from build123d import *

# Parameters (mm, degrees)
SKETCH1_R           = 10.5
SKETCH1_R_2         = 9
BOSS_EXTRUDE1_DEPTH = 15
CUT_EXTRUDE1_START  = 9.5
CUT_EXTRUDE1_DEPTH  = 2


with BuildPart() as part:
    # Sketch1 → Boss-Extrude1 (new body, symmetric)
    with BuildSketch(Plane(origin=(0, 0, 0), x_dir=(1, 0, 0), z_dir=(0, 1, 0))):
        Circle(SKETCH1_R)
        Circle(SKETCH1_R_2, mode=Mode.SUBTRACT)
    extrude(amount=BOSS_EXTRUDE1_DEPTH, both=True)

    # Sketch2 → Cut-Extrude1 (cut)
    with BuildSketch(Plane(origin=(0, 0, 0), x_dir=(0, 0, -1), z_dir=(1, 0, 0)).offset(CUT_EXTRUDE1_START)):
        with BuildLine():
            ThreePointArc((-2.374052789, 1.874699538), (-1.648827359, 2.536137485), (-0.75, 2.93055029))
            Line((-0.75, 2.93055029), (-0.75, 5))
            add(Edge.make_bspline(
                [(-0.75, 5), (-0.968656254, 3.654443702), (-2.374052789, 1.874699538)],
                knots=[0, 0, 0, 1, 1, 1], degree=2))
        make_face()
        with BuildLine():
            ThreePointArc((-2.374052789, -1.874699538), (-1.648827359, -2.536137485), (-0.75, -2.93055029))
            Line((-0.75, -2.93055029), (-0.75, 2.93055029))
            ThreePointArc((-0.75, 2.93055029), (-1.648827359, 2.536137485), (-2.374052789, 1.874699538))
            ThreePointArc((-2.374052789, 1.874699538), (-3.025, 0), (-2.374052789, -1.874699538))
        make_face()
        with BuildLine():
            Line((0.75, 2.93055029), (0.75, -2.93055029))
            ThreePointArc((0.75, -2.93055029), (1.648827359, -2.536137485), (2.374052789, -1.874699538))
            ThreePointArc((2.374052789, -1.874699538), (2.857633171, -0.992248788), (3.025, 0))
            ThreePointArc((3.025, 0), (2.857633171, 0.992248788), (2.374052789, 1.874699538))
            ThreePointArc((2.374052789, 1.874699538), (1.648827359, 2.536137485), (0.75, 2.93055029))
        make_face()
        with BuildLine():
            Line((0.75, 5), (0.75, 2.93055029))
            ThreePointArc((0.75, 2.93055029), (1.648827359, 2.536137485), (2.374052789, 1.874699538))
            add(Edge.make_bspline(
                [(0.75, 5), (0.968656254, 3.654443702), (2.374052789, 1.874699538)],
                knots=[0, 0, 0, 1, 1, 1], degree=2))
        make_face()
        with BuildLine():
            Line((0.75, -2.93055029), (0.75, -5))
            add(Edge.make_bspline(
                [(0.75, -5), (0.968656254, -3.654443702), (2.374052789, -1.874699538)],
                knots=[0, 0, 0, 1, 1, 1], degree=2))
            ThreePointArc((2.374052789, -1.874699538), (1.648827359, -2.536137485), (0.75, -2.93055029))
        make_face()
        with BuildLine():
            Line((-0.75, -5), (0.75, -5))
            Line((0.75, -5), (0.75, -2.93055029))
            ThreePointArc((0.75, -2.93055029), (0, -3.025), (-0.75, -2.93055029))
            Line((-0.75, -2.93055029), (-0.75, -5))
        make_face()
        with BuildLine():
            add(Edge.make_bspline(
                [(-0.75, -5), (-0.968656254, -3.654443702), (-2.374052789, -1.874699538)],
                knots=[0, 0, 0, 1, 1, 1], degree=2))
            Line((-0.75, -5), (-0.75, -2.93055029))
            ThreePointArc((-0.75, -2.93055029), (-1.648827359, -2.536137485), (-2.374052789, -1.874699538))
        make_face()
        with BuildLine():
            ThreePointArc((-0.75, 2.93055029), (0, 3.025), (0.75, 2.93055029))
            Line((0.75, 2.93055029), (0.75, 5))
            Line((0.75, 5), (-0.75, 5))
            Line((-0.75, 5), (-0.75, 2.93055029))
        make_face()
        with BuildLine():
            ThreePointArc((-0.75, -2.93055029), (0, -3.025), (0.75, -2.93055029))
            Line((0.75, -2.93055029), (0.75, 2.93055029))
            ThreePointArc((0.75, 2.93055029), (0, 3.025), (-0.75, 2.93055029))
            Line((-0.75, 2.93055029), (-0.75, -2.93055029))
        make_face()
    cut_extrude1 = extrude(amount=CUT_EXTRUDE1_DEPTH, mode=Mode.SUBTRACT)

    # Mirror1: Cut-Extrude1 across plane
    add(cut_extrude1.mirror(Plane(origin=(0, 0, 0), x_dir=(0, 0, 1), z_dir=(1, 0, 0))), mode=Mode.SUBTRACT)


solid = part.part
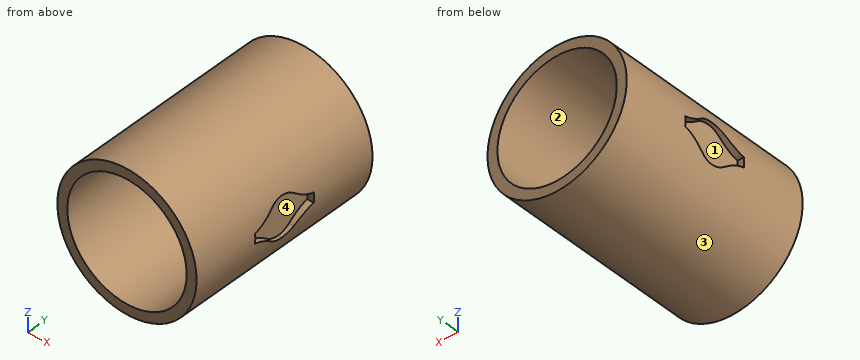
The listing builds one solid part. Answer for the finished solid, in the listing's coordinates (mm). Face numbers are marked on the shaded views. A direction names the side the tool comes from. Give positions to 0.01 mm unless a question says otherwise; leave off trailing zeros. Loops run counter-clockwise (first coordinate to the right, second up) from the corner with the lowest first, then second, coordinate; pieces in that order, holes last. Notation, with made-up numbers: (22, 13) - (52, 13) arc R31 cw to (52, 47) - close; hole circle Ø9 at (-39, -37.75). An arc over 180 degrees is marked (long way). Use one line per item in the form item = value.
1. Section C-C on y = -1 is taken. Give the vertices of the cut face in (x, z), then the cut area to 3 significant figures.
Calculated:
outline = (-10.1, -2.85) arc R10.5 ccw to (10.1, -2.85) - (9.5, -2.85) - (9.5, 2.85) - (10.1, 2.85) arc R10.5 ccw to (-10.1, 2.85) - (-9.5, 2.85) - (-9.5, -2.85) - close; hole circle Ø18 at (0, 0)
area = 82.0 mm^2
2. Which of the six approach directions +Z, -Z, +X, -X, +Y, -Y give full straight-line access (tool end or side, diameter ignored) to the marked faces 1 and 2?
Calculated:
face_1 = -X
face_2 = +Y, -Y
3. Find the intervals of material crossed by line 1 along X through (y, z) = (-0.25, 0); line 2 along X through (y, z) = (-5.5, 0); line 3 along Z through (x, y) = (2.5, -11), in increasing order. Write a range as [from, to].
Calculated:
line_1 = [-9.5, -9], [9, 9.5]
line_2 = [-10.5, -9], [9, 10.5]
line_3 = [-10.2, -8.65], [8.65, 10.2]
4. Section D-D on x = -4.25 is taken. Give the vertices of the cut face in (y, z), then the cut area to 3 significant figures.
Calculated:
outline = (-15, -9.6) - (15, -9.6) - (15, -7.93) - (-15, -7.93) - close; (-15, 7.93) - (15, 7.93) - (15, 9.6) - (-15, 9.6) - close
area = 100 mm^2
5. Section B-B on x = 0 is taken. Give the vertices of the cut face in (y, z), then the cut area to 3 significant figures.
Calculated:
outline = (-15, -10.5) - (15, -10.5) - (15, -9) - (-15, -9) - close; (-15, 9) - (15, 9) - (15, 10.5) - (-15, 10.5) - close
area = 90.0 mm^2
6. Section A-A on z = 0 is taken. Give the vertices of the cut face in (x, y).
Calculated:
outline = (-10.5, -15) - (-9, -15) - (-9, 15) - (-10.5, 15) - (-10.5, 5) - (-9.5, 5) - (-9.5, -5) - (-10.5, -5) - close; (9, -15) - (10.5, -15) - (10.5, -5) - (9.5, -5) - (9.5, 5) - (10.5, 5) - (10.5, 15) - (9, 15) - close
7. Given pin 1 Ø1 at (x, y) = (4, 2) entering from +Z; pin 2 Ø10 at (y, z) = (0.5, 3.5) entering from +X; pin 3 Ø5 at (x, y) = (-0.5, -9.5) entering from -Z; pin 4 Ø6.5 at (y, z) = (0, 0) entering from -X, each flat-ended and moving along its own axis, determine where each tip first touches the part or whether it passes through.
Calculated:
pin_1 = 9.9
pin_2 = 10.47
pin_3 = -10.5
pin_4 = -10.35
8. The mould has two halves that part along Z. Classify the marked faces 3 and 4: pulls with the +Z half, pulls with the -Z half, needs draft (parallel to the pull), parting line crosses it, or undercut.
Calculated:
face_3 = parting line crosses it
face_4 = undercut
